Part print with two shaded views. Sizes in mm from the minimum x, y, z corner. Round coordinates to 2 decimals unless told otherwise and drop trailing zeros. Write each loop counter-clockwise with the first axis right and the second up, starting at its lowest first coordinate (ties: lowest second). Pieces come first, ordered by that corner, then holes. Notation, with made-up numbers: (39.5, -10.75) -> (78.5, -10.75) arc R26 cw to (78.5, 5.25) -> close; hole circle Ø5 at (-29, -27). An arc over 180 degrees is marked (long way). Answer as CSV lines item,"result".
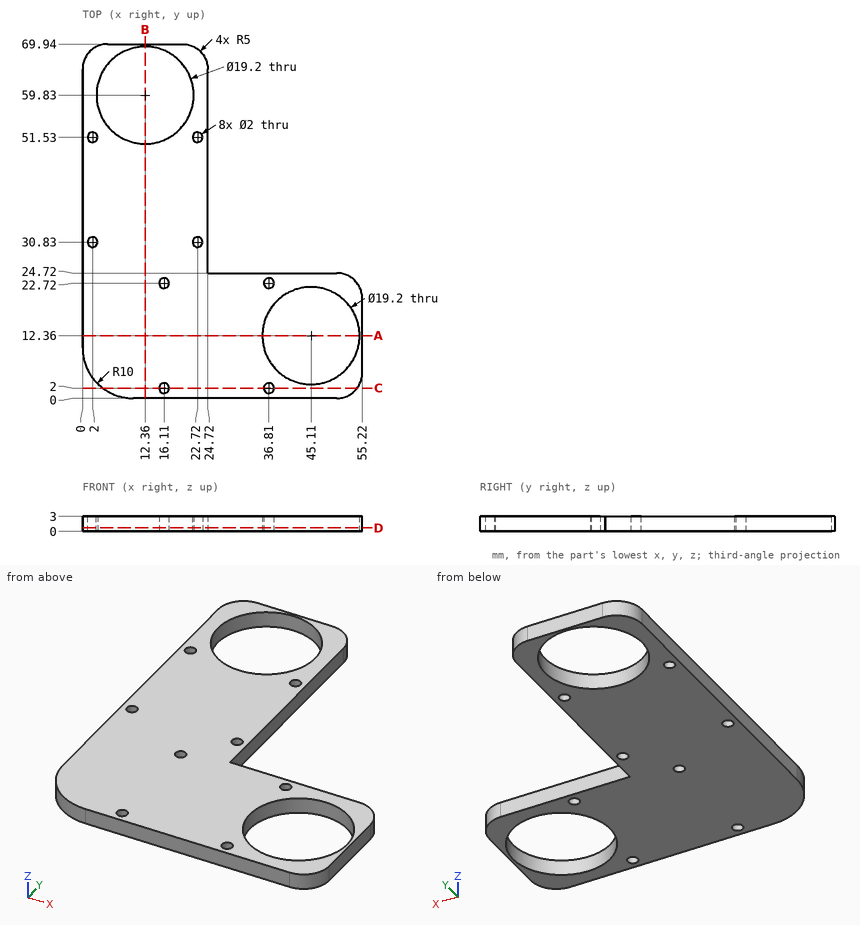
1. Cut at C-C, the plane y = 2. Write the cut outline in (x, z).
Results found:
outline,"(4, 0) -> (15.11, 0) -> (15.11, 3) -> (4, 3) -> close; (17.11, 0) -> (35.81, 0) -> (35.81, 3) -> (17.11, 3) -> close; (37.81, 0) -> (54.22, 0) -> (54.22, 3) -> (37.81, 3) -> close"
2. Cut at B-B, the plane x = 12.36. Write the cut outline in (y, z).
Results found:
outline,"(0, 0) -> (50.23, 0) -> (50.23, 3) -> (0, 3) -> close; (69.43, 0) -> (69.94, 0) -> (69.94, 3) -> (69.43, 3) -> close"
3. Cut at D-D, the plane z = 0.7. Count the separate pieces of the cut face and the enclosed holes in it, then the cut area to 3 significant figures.
Results found:
separate pieces,"1"
enclosed holes,"10"
area,"1,840 mm2"
4. Probe line 1 along Y through (x, z) = (45.11, 0.9); line 2 along Y through (x, z) = (2, 1.7); line 3 along Y through (x, z) = (15.5, 1.4). List the from-to ranges inside material, lowest first.
Results found:
line 1,"y = 0 to 2.76, 21.96 to 24.72"
line 2,"y = 4 to 29.83, 31.83 to 50.53, 52.53 to 68.94"
line 3,"y = 0 to 1.21, 2.79 to 21.93, 23.51 to 50.76, 68.9 to 69.94"
5. Cut at A-A, the plane y = 12.36. Write the cut outline in (x, z).
Results found:
outline,"(0, 0) -> (35.51, 0) -> (35.51, 3) -> (0, 3) -> close; (54.71, 0) -> (55.22, 0) -> (55.22, 3) -> (54.71, 3) -> close"
6. Drop a flat-ended pin along its axis: pin 1 Ø0.9 at (y, z) = (55, 1) entering from +X. Give the stop position or say it passes through.
Results found:
pin 1,"stops at x = 24.72"
